Geometry: final body of the model. Coordinates: model frame, mm. A direction names the side the tool comes from. Coordinates: 2 decimals unless noted, no trailing zeros. Order: outer loops, then holes, each group sorted by start corner. A loop starts at its lowest first (then second) coordinate and runs counter-clockwise, first axis right, second up. Notation, with made-up numbers: (15, -23) - (53, -23) arc R25 ccw to (53, 14) - close; hole circle Ø6 at (21.25, 76). An arc over 180 degrees is marked (long way). Use a Markdown table: item, result. Add a question column.
```python
from build123d import *

# Parameters (mm, degrees)
SKETCH2_W           = 20
SKETCH2_H           = 9
BOSS_EXTRUDE1_DEPTH = 8
SKETCH3_W           = 4
SKETCH3_H           = 5
CUT_EXTRUDE1_DEPTH  = 10
SKETCH6_W           = 20
SKETCH6_H           = 2
BOSS_EXTRUDE3_DEPTH = 40


with BuildPart() as part:
    # Sketch2 → Boss-Extrude1 (new body)
    with BuildSketch(Plane.XY):
        Rectangle(SKETCH2_W, SKETCH2_H)
    extrude(amount=BOSS_EXTRUDE1_DEPTH)

    # Sketch3 → Cut-Extrude1 (cut)
    with BuildSketch(Plane.ZY.offset(10)):
        with Locations((4, 0)):
            Rectangle(SKETCH3_W, SKETCH3_H)
    extrude(amount=-CUT_EXTRUDE1_DEPTH, mode=Mode.SUBTRACT)

    # Sketch6 → Boss-Extrude3 (add)
    with BuildSketch(Plane(origin=(0, 4.5, 0), x_dir=(1, 0, 0), z_dir=(0, 1, 0))):
        with Locations((0, -4)):
            Rectangle(SKETCH6_W, SKETCH6_H)
    extrude(amount=BOSS_EXTRUDE3_DEPTH)


solid = part.part
```
1) Section D-D (z = 7). Return loops of the section in (x, y), then the cut area to 3 significant figures.
2) Section C-C (y = 0.5). Return loops of the section in (x, z).
3) Section A-A (x = -7.25). Return loops of the section in (y, z).
4) Ray query, line 1 along Y through (x, z) = (-4.5, 5.5); line 2 along Y through (x, z) = (-5.5, 4.5); line 3 along Z through (x, y) = (2.75, 41.5). Return the intervals inside material, ascending.
5) Draft query along Y for faces 1 (the face through (10, 14, 4)), 2 (the face through (0, 0, 4)), 3 (the face through (0, -4.5, 4)). Return one class per face: pulls with the +Y half, pulls with the -Y half, needs draft (parallel to the pull), parting line crosses it, or undercut.
6) Pin query (flat end, axial travel): pin 1 (1 mm diameter, centred on x = 2, y = 13.5, fed in from -Z); pin 2 (3 mm diameter, centred on x = -0.5, z = 5.5, fed in from +Y); pin 3 (0.9 mm diameter, centred on x = -2, z = 6, fed in from +Y). Return the tip coordinate at first contact, or that it passes through.
7) Set-up query: faces 4 (the face through (0, 0, 8)), 5 (the face through (0, 24, 5)), 6 (the face through (0, 4.5, 1)), 7 (the face through (-5, 0, 6)), 8 (the face through (0, 44.5, 4)). Return all of +Z, -Z, +X, -X, +Y, -Y with unobstructed straight access to the full face (end or side cutting, diameter ignored); none if empty.
8) Section B-B (z = 4.25). Return loops of the section in (x, y), then the cut area to 3 significant figures.
Values follow:
| question | item | result |
|---|---|---|
| 1 | outline | (-10, -4.5) - (10, -4.5) - (10, 4.5) - (-10, 4.5) - close |
| 1 | area | 180 mm² |
| 2 | outline | (-10, 0) - (10, 0) - (10, 8) - (-10, 8) - (-10, 6) - (0, 6) - (0, 2) - (-10, 2) - close |
| 3 | outline | (-4.5, 0) - (4.5, 0) - (4.5, 3) - (44.5, 3) - (44.5, 5) - (4.5, 5) - (4.5, 8) - (-4.5, 8) - close; hole (-2.5, 2) - (2.5, 2) - (2.5, 6) - (-2.5, 6) - close |
| 4 | line 1 | y = -4.5 to -2.5, 2.5 to 4.5 |
| 4 | line 2 | y = -4.5 to -2.5, 2.5 to 44.5 |
| 4 | line 3 | z = 3 to 5 |
| 5 | face 1 | needs draft |
| 5 | face 2 | undercut |
| 5 | face 3 | pulls with the -Y half |
| 6 | pin 1 | stops at z = 3 |
| 6 | pin 2 | stops at y = 44.5 |
| 6 | pin 3 | stops at y = 4.5 |
| 7 | face 4 | +Z, +X, -X, +Y, -Y |
| 7 | face 5 | +Z, +X, -X, +Y |
| 7 | face 6 | -Z, +X, -X, +Y |
| 7 | face 7 | -X |
| 7 | face 8 | +Z, -Z, +X, -X, +Y |
| 8 | outline | (-10, -4.5) - (10, -4.5) - (10, 44.5) - (-10, 44.5) - (-10, 2.5) - (0, 2.5) - (0, -2.5) - (-10, -2.5) - close |
| 8 | area | 930 mm² |
